Check sheet for the modelled part. Datum: model origin and axes. Units: mm. Face numbers are marked on the shaded views. Give positions to 0.01 mm unless a question says otherwise; leave off trailing zeros. Order: outer loops, then holes, each group sorted by start corner. A loop starts at its lowest first (then second) coordinate and runs counter-clockwise, first axis right, second up.
```python
from build123d import *

# Parameters (mm, degrees)
SKETCH_1_W               = 20
SKETCH_1_H               = 20
SKETCH_1_W_2             = 18
SKETCH_1_H_2             = 18
EXTRUDE_1_DEPTH          = 83.5
CUT_EXTRUDE_2_DEPTH      = 85.689137438
CUT_EXTRUDE_2_DEPTH_BACK = 85.689137438
SKETCH_3_R               = 2
SKETCH_5_W               = 13
SKETCH_5_H               = 20
CUT_EXTRUDE_3_DEPTH      = 87.442177205
SKETCH_7_R               = 2
CUT_EXTRUDE_4_DEPTH      = 87.442177205


with BuildPart() as part:
    # 草图1 → 凸台-拉伸1 (new, symmetric)
    with BuildSketch(Plane.XY):
        Rectangle(SKETCH_1_W, SKETCH_1_H)
        Rectangle(SKETCH_1_W_2, SKETCH_1_H_2, mode=Mode.SUBTRACT)
    extrude(amount=EXTRUDE_1_DEPTH, both=True)

    # 草图3 → 切除-拉伸2 (cut, two sides: drawn at the far end of the back side and taken through both)
    with BuildSketch(Plane(origin=(0, 0, 0), x_dir=(1, 0, 0), z_dir=(0, 1, 0)).offset(-CUT_EXTRUDE_2_DEPTH_BACK)):
        with Locations(Location((0.645896247, -30.788728887, 0), (0, 0, 270))):
            Circle(SKETCH_3_R)
        with Locations(Location((0.645896247, -10.788728887, 0), (0, 0, 270))):
            Circle(SKETCH_3_R)
        with Locations(Location((0.645896247, 36.711271113, 0), (0, 0, 270))):
            Circle(SKETCH_3_R)
        with Locations(Location((0.645896247, 45.211271113, 0), (0, 0, 270))):
            Circle(SKETCH_3_R)
        with Locations(Location((0.645896247, 65.211271113, 0), (0, 0, 270))):
            Circle(SKETCH_3_R)
    extrude(amount=CUT_EXTRUDE_2_DEPTH + CUT_EXTRUDE_2_DEPTH_BACK, mode=Mode.SUBTRACT)

    # 草图5 → 切除-拉伸3 (cut, through all)
    with BuildSketch(Plane(origin=(10, 0, 0), x_dir=(0, 0, -1), z_dir=(1, 0, 0))):
        with Locations((77, 0)):
            Rectangle(SKETCH_5_W, SKETCH_5_H)
    extrude(amount=-CUT_EXTRUDE_3_DEPTH, mode=Mode.SUBTRACT)

    # 草图7 → 切除-拉伸4 (cut, through all)
    with BuildSketch(Plane(origin=(10, 0, 0), x_dir=(0, 0, -1), z_dir=(1, 0, 0))):
        with Locations(Location((55.5, 0, 0), (0, 0, 90))):
            Circle(SKETCH_7_R)
    extrude(amount=-CUT_EXTRUDE_4_DEPTH, mode=Mode.SUBTRACT)


solid = part.part
```
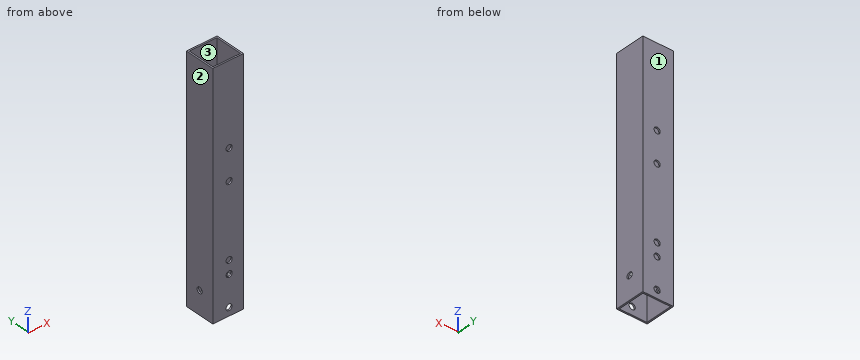
(1) Cross-section at A-A on y = 4. Enter the section's corners in (x, z), then the cut area to 3 significant figures.
Response values:
outline: (-10, -70.5) - (-9, -70.5) - (-9, 83.5) - (-10, 83.5) - close; (9, -70.5) - (10, -70.5) - (10, 83.5) - (9, 83.5) - close
area: 308 mm2
(2) Cross-section at B-B on z = -60. Enter the section's corners in (x, y).
Response values:
outline: (-10, -10) - (10, -10) - (10, 10) - (-10, 10) - close; hole (-9, -9) - (9, -9) - (9, 9) - (-9, 9) - close
(3) Release check for a two-part mould opening along X. For the marked faces 1, 2 and 3 record: released by +X, released by -X, zero draft, split by the parting line, or undercut.
Response values:
face 1: zero draft
face 2: released by -X
face 3: undercut
(4) Material ranges on L1, parallel to X at y = -8.25, z = -1; L2, parallel to Z at x = -9.55, y = 0, recorded low to high.
Response values:
L1: x = -10 to -9, 9 to 10
L2: z = -70.5 to -57.5, -53.5 to 83.5
